```python
from build123d import *

# Parameters (mm, degrees)
F0_R     = 6
F1_DEPTH = 40
F0_R_2   = 10
F0_W     = 140
F0_H     = 140
F2_DEPTH = 15


with BuildPart() as f1:
    # F0 (on Front) → F1 (new body)
    with BuildSketch(Plane.XZ):
        with Locations((-49.8, 0)):
            Circle(F0_R)
    extrude(amount=F1_DEPTH)



with BuildPart() as f1b:
    # F0 (on Front) → F1, piece 2 (new body)
    with BuildSketch(Plane.XZ):
        Circle(F0_R_2)
    extrude(amount=F1_DEPTH)


with BuildPart() as f1_1:
    add(f1.part)

    add(f1b.part)  # F2 merges F1b
    # F0 (on Front) → F2 (join)
    with BuildSketch(Plane.XZ):
        Rectangle(F0_W, F0_H)
        with Locations((-49.8, 0)):
            Circle(F0_R, mode=Mode.SUBTRACT)
        Circle(F0_R_2, mode=Mode.SUBTRACT)
    extrude(amount=F2_DEPTH)


solid = f1_1.part
```
Build history of the part. All positions in model axes, mm. A direction names the side the tool comes from. Coordinates: 2 decimals unless noted, no trailing zeros. Order: outer loops, then holes, each group sorted by start corner. A loop starts at its lowest first (then second) coordinate and runs counter-clockwise, first axis right, second up. Notation, with made-up numbers: (70.5, 7.25) -> (77.5, 7.25) arc R37 cw to (77.5, 43.25) -> close; hole circle Ø5 at (-17, 89). An arc over 180 degrees is marked (long way). Answer in a Markdown table with one row per item. Add a question column.
Q1. Mould opens along X. For faces 3 (the face through (-70, -7, -1)), 4 (the face through (-44.26, -27.32, -2.3)), 5 (the face through (-1, -7, 70)), 6 (the face through (70, -7, -1)) say: +X half, -X half, draft (parallel to the pull), parting line (faces both ways), or undercut.
Q2. Band-saw the part on D-D, the plane x = -49.8. List the corners of the cut face in (y, z).
Q3. Band-saw the part on C-C, the plane z = 0. List the corners of the cut face in (x, y).
Q4. Band-saw the part on B-B, the plane y = -19.5. List the corners of the cut face in (x, z).
Q5. Which spindle directions (+Z, -Z, +X, -X, +Y, -Y) get a long thin tool onto all of the face, cutting with end or side? Do faces 1 (the face through (-2.17, -27.32, -9.76)), 2 (the face through (-50, -40, 0)). Say none if no direction does.
Q6. Band-saw the part on A-A, the plane x = 0. List the corners of the cut face in (y, z), then the cut area to 3 significant figures.
Q7. Wall check: line 1 along Y through (x, z) = (-44.5, -61.5); line 2 along X through (y, z) = (-22, 7.5). Give the ranges that are in metal, low to high. Write a range as [from, to].
Answers follow:
| question | item | result |
|---|---|---|
| 1 | face 3 | -X half |
| 1 | face 4 | undercut |
| 1 | face 5 | draft |
| 1 | face 6 | +X half |
| 2 | outline | (-40, -6) -> (-15, -6) -> (-15, -70) -> (0, -70) -> (0, 70) -> (-15, 70) -> (-15, 6) -> (-40, 6) -> close |
| 3 | outline | (-70, -15) -> (-55.8, -15) -> (-55.8, -40) -> (-43.8, -40) -> (-43.8, -15) -> (-10, -15) -> (-10, -40) -> (10, -40) -> (10, -15) -> (70, -15) -> (70, 0) -> (-70, 0) -> close |
| 4 | outline | circle Ø12 at (-49.8, 0); circle Ø20 at (0, 0) |
| 5 | face 1 | -Y |
| 5 | face 2 | +Z, -Z, +X, -X, -Y |
| 6 | outline | (-40, -10) -> (-15, -10) -> (-15, -70) -> (0, -70) -> (0, 70) -> (-15, 70) -> (-15, 10) -> (-40, 10) -> close |
| 6 | area | 2,600 mm^2 |
| 7 | line 1 | [-15, 0] |
| 7 | line 2 | [-6.61, 6.61] |
